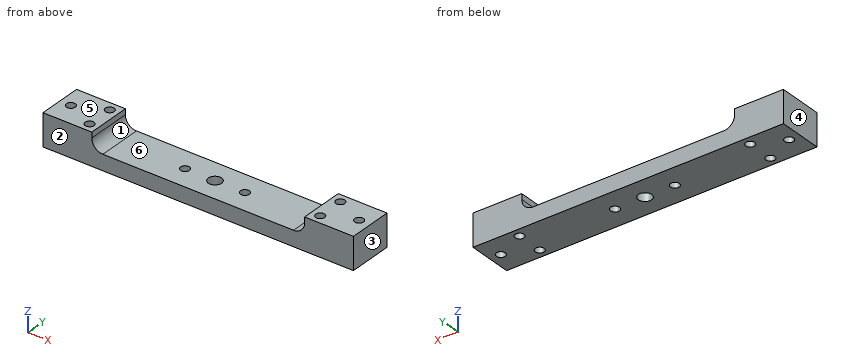
Autodesk Inventor part; units mm, degrees
ref_plane "YZ Plane" through (0, 0, 0) normal (1, 0, 0) x (0, 1, 0)
ref_plane "XZ Plane" through (0, 0, 0) normal (0, 1, 0) x (-1, 0, 0)
ref_plane "XY Plane" through (0, 0, 0) normal (0, 0, 1) x (1, 0, 0)
sketch "Sketch1" plane through (0, 0, 0) normal (0, 0, 1) x (1, 0, 0)
  line L0 (-70, 10) -> (70, 10)
  line L1 (70, 10) -> (70, -10)
  line L2 (70, -10) -> (-70, -10)
  line L3 (-70, -10) -> (-70, 10)
  line L4 (-70, 10) -> (70, -10) construction
  line L5 (70, 10) -> (-70, -10) construction
  line L6 (0, 0) -> (-13.5, 0) construction
  line L7 (-13.5, 0) -> (13.5, 0) construction
  circle A0 centre (-13.5, 0) radius 2
  circle A1 centre (13.5, 0) radius 2
  circle A2 centre (0, 0) radius 3
  dimension "d0" = 140
  dimension "d1" = 20
  dimension "d2" = 13.5
  dimension "d3" = 27
  dimension "d4" = 4
  dimension "d5" = 4
  dimension "d6" = 6
extrude "Extrusion1" add sketch "Sketch1" along normal mid plane 7
sketch "Sketch2" plane through (-70, -10, 3.5) normal (0, -1, 0) x (1, 0, 0)
  line L0 (70, -3.5) -> (30, -3.5) construction
  line L1 (30, -3.5) -> (110, -3.5) construction
  line L2 (0, 0) -> (140, 0)
  line L3 (22, 5) -> (22, 7.5)
  line L4 (22, 7.5) -> (2, 7.5)
  line L5 (0, 5.5) -> (0, 0)
  line L6 (0, 0) -> (22, 0)
  line L7 (70, -9.525) -> (70, 0) construction
  line L8 (27, 0) -> (140, 0)
  arc A0 (22, 5) -> (27, 0) centre (27, 5) ccw
  line L9 (27, 0) -> (22, 0)
  line L10 (140, 0) -> (0, 0)
  line L11 (118, 5) -> (118, 7.5)
  line L12 (118, 7.5) -> (138, 7.5)
  line L13 (140, 5.5) -> (140, 0)
  arc A1 (113, 0) -> (118, 5) centre (113, 5) ccw
  line L14 (140, 5.5) -> (140, 7.5)
  line L15 (140, 7.5) -> (138, 7.5)
  line L16 (0, 5.5) -> (0, 7.5)
  line L17 (0, 7.5) -> (2, 7.5)
  point P0 (113, 0)
  dimension "d13" = 40
  dimension "d14" = 80
  dimension "d15" = 7.5
  dimension "d16" = 5
extrude "Extrusion2" add sketch "Sketch2" against normal blind 20
sketch "Sketch3" plane through (48, -10, 11) normal (0, 0, 1) x (1, 0, 0)
  line L0 (-48, 10) -> (12, 10) construction
  line L1 (12, 10) -> (17, 10) construction
  circle A0 centre (17, 10) radius 2
  line L2 (12, 10) -> (4, 10) construction
  line L3 (4, 10) -> (4, 4) construction
  line L4 (4, 4) -> (4, 16) construction
  circle A1 centre (4, 4) radius 2
  circle A2 centre (4, 16) radius 2
  line L5 (-48, 10) -> (-48, 19.9246) construction
  circle A3 centre (-113, 10) radius 2
  circle A4 centre (-100, 4) radius 2
  circle A5 centre (-100, 16) radius 2
  dimension "d20" = 60
  dimension "d21" = 5
  dimension "d22" = 4
  dimension "d23" = 8
  dimension "d24" = 6
  dimension "d25" = 12
  dimension "d26" = 4
  dimension "d27" = 4
extrude "Extrusion3" cut sketch "Sketch3" against normal blind 17.5
equation "\"BendRadius\" = Thickness"
equation "\"BendReliefWidth\" = Thickness"
equation "\"BendReliefDepth\" = 0.5 * Thickness"
equation "\"CornerReliefSize\" = 4 * Thickness"
equation "\"MinimumRemnant\" = 2 * Thickness"
equation "\"TransitionRadius\" = BendRadius"
equation "\"JacobiRadiusSize\" = BendRadius"
equation "\"GapSize\" = Thickness"
properties part number "Uchwyt na ramę" material "Steel"
Check sheet for the modelled part. Datum: model origin and axes. Units: mm. Face numbers are marked on the shaded views. A direction names the side the tool comes from. Coordinates: 2 decimals unless noted, no trailing zeros. Order: outer loops, then holes, each group sorted by start corner. A loop starts at its lowest first (then second) coordinate and runs counter-clockwise, first axis right, second up. Notation, with made-up numbers: (-28, -32.5) -> (9, -32.5) arc R19 ccw to (9, -23.5) -> close; hole circle Ø6 at (16.25, 19.25). An arc over 180 degrees is marked (long way). Write each question's results on one line, items separated by ' | '. Start each with the question number.
1) Section check D-D (z = -1.5). Count the separate pieces of the cut face and the enclosed holes in it, and give its area (3 significant figures).
2) Draft check along X on the marked faces 3, 4, 5 and 6. Enter one of: pulls with the +X half, pulls with the -X half, needs draft (parallel to the pull), parting line crosses it, or undercut.
3) Section check A-A (z = 9.75). Enter the section's corners in (x, y), and give its area (3 significant figures).
4) Section check B-B (x = -52). Enter the section's corners in (y, z).
5) Material ranges on line 1 along Y through (x, z) = (-52, 6); line 2 along X through (y, z) = (7.75, 4.25); line 3 along Z through (x, y) = (-16.5, -4), recorded low to high.
6) Depth check by flat-ended pin: pin 1 (5.5 mm diameter, centred on x = 0, y = 0, fed in from +Z); pin 2 (3 mm diameter, centred on x = 24.5, y = 3.5, fed in from +Z). Enter the tip coordinate at first touch or a pass-through.
7) Set-up check for the marked faces 1 and 2: record each of +Z, -Z, +X, -X, +Y, -Y from which the full face is reachable in a straight line by a thin tool's end or side.
8) Section check C-C (x = -13.5). Enter the section's corners in (y, z).
Checked values:
1) separate pieces: 1 | enclosed holes: 9 | area: 2,670 mm²
2) face 3: pulls with the +X half | face 4: pulls with the -X half | face 5: needs draft | face 6: undercut
3) outline: (-70, -10) -> (-48, -10) -> (-48, 10) -> (-70, 10) -> close; (48, -10) -> (70, -10) -> (70, 10) -> (48, 10) -> close; hole circle Ø4 at (-65, 0); hole circle Ø4 at (-52, -6); hole circle Ø4 at (-52, 6); hole circle Ø4 at (52, -6); hole circle Ø4 at (52, 6); hole circle Ø4 at (65, 0) | area: 805 mm²
4) outline: (-10, -3.5) -> (-8, -3.5) -> (-8, 11) -> (-10, 11) -> close; (-4, -3.5) -> (4, -3.5) -> (4, 11) -> (-4, 11) -> close; (8, -3.5) -> (10, -3.5) -> (10, 11) -> (8, 11) -> close
5) line 1: -10 to -8, -4 to 4, 8 to 10 | line 2: -70 to -52.97, -51.03 to -45.63, 45.63 to 51.03, 52.97 to 70 | line 3: -3.5 to 3.5
6) pin 1: through | pin 2: z = 3.5
7) face 1: +Z, +Y, -Y | face 2: +Z, -Z, +X, -X, -Y
8) outline: (-10, -3.5) -> (-2, -3.5) -> (-2, 3.5) -> (-10, 3.5) -> close; (2, -3.5) -> (10, -3.5) -> (10, 3.5) -> (2, 3.5) -> close
